Work out the finished part from the listing and answer in its coordinate system (mm). A direction names the side the tool comes from. Coordinates: 2 decimals unless noted, no trailing zeros. Write each loop counter-clockwise with the first axis right and the second up, starting at its lowest first coordinate (ties: lowest second). Pieces come first, ordered by that corner, then holes. Notation, with made-up numbers: (69, -15.5) - (87, -15.5) arc R14 ccw to (87, -9.5) - close; hole circle Ø3 at (-24, -15). An arc over 180 degrees is marked (long way). Use a Markdown table: item, result. Add a question column.
(1) A tool of negligible diameter and unlimited length cuts with its end or side. For faces 1 (the face through (-76, 0, 3)), 2 (the face through (-42, 22.7, 3)), 3 (the face through (-22, 39, 3)), 4 (the face through (-79, 23, 3)), 5 (the face through (-43, 17, 0)), from which of +Z, -Z, +X, -X, +Y, -Y can it reach the whole face along a straight path? Write none if from no direction.
(2) The part is cut by section B-B, the plane x = -75. Give the vertices of the cut face in (y, z), then the cut area to 3 significant figures.
(3) Find the intervals of material crossed by line 1 (Y direction, x = -9, z = 4.2); line 2 (X direction, y = 19, z = 0.8); line 3 (X direction, y = 26.5, z = 2.55), in increasing order. Write a range as from..to.
(4) Given pin 1 Ø0.8 at (x, z) = (-44.5, 3) entering from +Y; pin 2 Ø3 at (x, z) = (-67, 2) entering from -Y; pin 3 Ø1.8 at (x, z) = (-14.5, 2) entering from -Y; pin 4 Ø1.8 at (x, y) = (-9, 34.5) entering from +Z, each flat-ended and moving along its own axis, determine where each tip first touches the part or whether it passes through.
(5) For a pull along X with two mould halves and no side action, classify faces 6 (the face through (-43.5, 32, 3)), 7 (the face through (-43, 17, 6)), 8 (the face through (-82.289, 37.196, 2.958)) as released by +X, released by -X, zero draft, split by the parting line, or undercut.
(6) The part is cut by section A-A, the plane y = 6. Give the vertices of the cut face in (x, z).
(7) The part is cut by section D-D, the plane x = -3. Give the vertices of the cut face in (y, z), then the cut area to 3 significant figures.
(8) The part is cut by section C-C, the plane y = 11. Give the vertices of the cut face in (x, z), then the cut area to 3 significant figures.
Autodesk Inventor part; units mm, degrees
ref_plane "YZ Plane" through (0, 0, 0) normal (1, 0, 0) x (0, 1, 0)
ref_plane "XZ Plane" through (0, 0, 0) normal (0, 1, 0) x (-1, 0, 0)
ref_plane "XY Plane" through (0, 0, 0) normal (0, 0, 1) x (1, 0, 0)
sketch "Sketch1" plane through (0, 0, 0) normal (0, 0, 1) x (1, 0, 0)
  arc A0 (-78, 39) -> (-84, 33) centre (-78, 33) ccw
  line L0 (-84, 33) -> (-84, 4)
  arc A1 (-84, 4) -> (-80, 0) centre (-80, 4) ccw
  line L1 (-80, 0) -> (-72, 0)
  arc A2 (-68.2919, -2.5) -> (-72, 0) centre (-72, -4) ccw
  arc A3 (-68.2919, -2.5) -> (-64.5838, -5) centre (-64.5838, -1) ccw
  line L2 (-64.5838, -5) -> (-45.4162, -5)
  arc A4 (-45.4162, -5) -> (-41.7081, -2.5) centre (-45.4162, -1) ccw
  arc A5 (-38, 0) -> (-41.7081, -2.5) centre (-38, -4) ccw
  line L3 (-38, 0) -> (-4, 0)
  arc A6 (-4, 0) -> (0, 4) centre (-4, 4) ccw
  line L4 (0, 4) -> (0, 33)
  arc A7 (0, 33) -> (-6, 39) centre (-6, 33) ccw
  line L5 (-6, 39) -> (-39, 39)
  line L6 (-39, 39) -> (-39, 33)
  line L7 (-39, 33) -> (-40.5, 33)
  line L8 (-40.5, 33) -> (-40.5, 30.5)
  line L9 (-40.5, 30.5) -> (-39.25, 30.5)
  line L10 (-39.25, 30.5) -> (-39.25, 28.7)
  line L11 (-39.25, 28.7) -> (-40.5, 28.7)
  line L12 (-40.5, 28.7) -> (-40.5, 22.7)
  line L13 (-40.5, 22.7) -> (-43.5, 22.7)
  line L14 (-43.5, 22.7) -> (-43.5, 28.7)
  line L15 (-43.5, 28.7) -> (-44.75, 28.7)
  line L16 (-44.75, 28.7) -> (-44.75, 30.5)
  line L17 (-44.75, 30.5) -> (-43.5, 30.5)
  line L18 (-43.5, 30.5) -> (-43.5, 33)
  line L19 (-43.5, 33) -> (-45, 33)
  line L20 (-45, 33) -> (-45, 39)
  line L21 (-45, 39) -> (-78, 39)
  line L22 (-63, -3.5) -> (-63, 16.5)
  line L23 (-63, 16.5) -> (-47, 16.5)
  line L24 (-47, 16.5) -> (-47, -3.5)
  line L25 (-47, -3.5) -> (-63, -3.5)
  line L26 (-79, 18.2) -> (-79, 28.8)
  line L27 (-79, 28.8) -> (-55, 28.8)
  line L28 (-55, 28.8) -> (-55, 18.2)
  line L29 (-55, 18.2) -> (-79, 18.2)
  line L30 (-29, 18.2) -> (-29, 28.8)
  line L31 (-29, 28.8) -> (-5, 28.8)
  line L32 (-5, 28.8) -> (-5, 18.2)
  line L33 (-5, 18.2) -> (-29, 18.2)
  circle A8 centre (-66, 6) radius 1.5
  circle A9 centre (-44, 6) radius 1.5
  circle A10 centre (-3, 3) radius 1.5
  circle A11 centre (-81, 3) radius 1.5
  circle A12 centre (-75, 34.5) radius 1.5
  circle A13 centre (-9, 34.5) radius 1.5
  point P0 (0, 0)
  point P1 (0, 0)
extrude "Extrusion1" add sketch "Sketch1" along normal blind 6
properties part number "XcrLeft_a"
Model answer:
| question | item | result |
|---|---|---|
| 1 | face 1 | +Z, -Z, -X, -Y |
| 1 | face 2 | +Z, -Z, +Y |
| 1 | face 3 | +Z, -Z, +X, -X, +Y |
| 1 | face 4 | +Z, -Z |
| 1 | face 5 | -Z, +X, -X, +Y, -Y |
| 2 | outline | (0, 0) - (18.2, 0) - (18.2, 6) - (0, 6) - close; (28.8, 0) - (33, 0) - (33, 6) - (28.8, 6) - close; (36, 0) - (39, 0) - (39, 6) - (36, 6) - close |
| 2 | area | 152 mm^2 |
| 3 | line 1 | 0..18.2, 28.8..33, 36..39 |
| 3 | line 2 | -84..-79, -55..-29, -5..0 |
| 3 | line 3 | -84..-79, -55..-43.5, -40.5..-29, -5..0 |
| 4 | pin 1 | y = 33 |
| 4 | pin 2 | y = -4.89 |
| 4 | pin 3 | y = 0 |
| 4 | pin 4 | through |
| 5 | face 6 | undercut |
| 5 | face 7 | zero draft |
| 5 | face 8 | released by -X |
| 6 | outline | (-84, 0) - (-67.5, 0) - (-67.5, 6) - (-84, 6) - close; (-64.5, 0) - (-63, 0) - (-63, 6) - (-64.5, 6) - close; (-47, 0) - (-45.5, 0) - (-45.5, 6) - (-47, 6) - close; (-42.5, 0) - (0, 0) - (0, 6) - (-42.5, 6) - close |
| 7 | outline | (0.13, 0) - (1.5, 0) - (1.5, 6) - (0.13, 6) - close; (4.5, 0) - (38.2, 0) - (38.2, 6) - (4.5, 6) - close |
| 7 | area | 210 mm^2 |
| 8 | outline | (-84, 0) - (-63, 0) - (-63, 6) - (-84, 6) - close; (-47, 0) - (0, 0) - (0, 6) - (-47, 6) - close |
| 8 | area | 408 mm^2 |
